from build123d import *

# Parameters (mm, degrees)
SKETCH1_W            = 350
SKETCH1_H            = 250
SKETCH1_W_2          = 329.63
SKETCH1_H_2          = 229.64
BOSS_EXTRUDE2_DEPTH  = 30
SKETCH1_3_W          = 329.63
SKETCH1_3_H          = 229.64
BOSS_EXTRUDE3_DEPTH  = 3.3
FILLET1_R            = 10
SKETCH3_W            = 40
SKETCH3_H            = 60
BOSS_EXTRUDE4_DEPTH  = 10
FILLET3_R            = 10
FILLET4_R            = 10
FILLET3_OF_MIRROR3_R = 10
FILLET4_OF_MIRROR3_R = 10
FILLET5_START        = 25.0000001
FILLET5_DEPTH        = 4.9999999
FILLET5_START_2      = 14.9999999
FILLET5_2_DEPTH      = 10.0000002
FILLET5_START_3      = -155
FILLET5_3_DEPTH      = 310


with BuildPart() as part:
    # Sketch1 → Boss-Extrude2 (new body)
    with BuildSketch(Plane(origin=(0, 0, 0), x_dir=(1, 0, 0), z_dir=(0, 1, 0))):
        Rectangle(SKETCH1_W, SKETCH1_H)
        Rectangle(SKETCH1_W_2, SKETCH1_H_2, mode=Mode.SUBTRACT)
    extrude(amount=BOSS_EXTRUDE2_DEPTH)

    # Sketch1<3> → Boss-Extrude3 (add)
    with BuildSketch(Plane(origin=(0, 0, 0), x_dir=(1, 0, 0), z_dir=(0, 1, 0))):
        Rectangle(SKETCH1_3_W, SKETCH1_3_H)
    extrude(amount=BOSS_EXTRUDE3_DEPTH)

    # Fillet1
    fillet1_edges = [part.edges().sort_by_distance(p)[0] for p in [
        (0, 0, -125),
        (175, 0, 0),
        (0, 0, 125),
        (-175, 0, 0),
        (-175, 15, -125),
        (175, 15, -125),
        (175, 15, 125),
        (-175, 15, 125),
    ]]
    fillet(fillet1_edges, radius=FILLET1_R)

    # Sketch3 → Boss-Extrude4 (add)
    with BuildSketch(Plane.XY.offset(125)):
        with Locations((-124.4, 45)):
            Rectangle(SKETCH3_W, SKETCH3_H)
    boss_extrude4 = extrude(amount=BOSS_EXTRUDE4_DEPTH)

    # Fillet3
    fillet3_edges = [part.edges().sort_by_distance(p)[0] for p in [
        (-124.4, 15, 135),
    ]]
    fillet(fillet3_edges, radius=FILLET3_R - 0.0001)  # a hair under: the kernel refuses the full size

    # Fillet4
    fillet4_edges = [part.edges().sort_by_distance(p)[0] for p in [
        (-124.4, 75, 135),
        (-104.4, 75, 130),
        (-144.4, 75, 130),
    ]]
    fillet(fillet4_edges, radius=FILLET4_R - 0.0001)  # a hair under: the kernel refuses the full size

    # Mirror3: Boss-Extrude4 across plane
    add(boss_extrude4.mirror(Plane.XY))

    # Fillet3 of Mirror3
    fillet3_of_mirror3_edges = [part.edges().sort_by_distance(p)[0] for p in [
        (-124.4, 15, -135),
    ]]
    fillet(fillet3_of_mirror3_edges, radius=FILLET3_OF_MIRROR3_R - 0.0001)  # a hair under: the kernel refuses the full size

    # Fillet4 of Mirror3
    fillet4_of_mirror3_edges = [part.edges().sort_by_distance(p)[0] for p in [
        (-124.4, 75, -135),
        (-104.4, 75, -130),
        (-144.4, 75, -130),
    ]]
    fillet(fillet4_of_mirror3_edges, radius=FILLET4_OF_MIRROR3_R - 0.0001)  # a hair under: the kernel refuses the full size

    # Mirror4: read off the stored shape, not the designer's step
    # Mirror4: part across plane


with BuildPart() as part_1:
    add(part.part)
    add(part.part.mirror(Plane(origin=(0, 0, 0), x_dir=(0, 0, 1), z_dir=(1, 0, 0))))

    # Fillet5: read off the stored shape, not the designer's step
    # Fillet5 outline → Fillet5 (add)
    with BuildSketch(Plane(origin=(0, 0, 0), x_dir=(1, 0, 0), z_dir=(0, 1, 0)).offset(FILLET5_START)):
        with BuildLine():
            Line((104.4, 125), (104.4, 135))
            ThreePointArc((104.4, 135), (101.471067812, 127.928932188), (94.4, 125))
            Line((94.4, 125), (104.4, 125))
        make_face()
        with BuildLine():
            Line((144.4, 135), (144.4, 125))
            Line((144.4, 125), (154.4, 125))
            ThreePointArc((154.4, 125), (147.328932188, 127.928932188), (144.4, 135))
        make_face()
        with BuildLine():
            Line((-154.4, 125), (-144.4, 125))
            Line((-144.4, 125), (-144.4, 135))
            ThreePointArc((-144.4, 135), (-147.328932188, 127.928932188), (-154.4, 125))
        make_face()
        with BuildLine():
            Line((-104.4, 125), (-94.4, 125))
            ThreePointArc((-94.4, 125), (-101.471067812, 127.928932188), (-104.4, 135))
            Line((-104.4, 135), (-104.4, 125))
        make_face()
        with BuildLine():
            Line((-144.4, -135), (-144.4, -125))
            Line((-144.4, -125), (-154.4, -125))
            ThreePointArc((-154.4, -125), (-147.328932188, -127.928932188), (-144.4, -135))
        make_face()
        with BuildLine():
            ThreePointArc((-104.4, -135), (-101.471067812, -127.928932188), (-94.4, -125))
            Line((-94.4, -125), (-104.4, -125))
            Line((-104.4, -125), (-104.4, -135))
        make_face()
        with BuildLine():
            Line((154.4, -125), (144.4, -125))
            Line((144.4, -125), (144.4, -135))
            ThreePointArc((144.4, -135), (147.328932188, -127.928932188), (154.4, -125))
        make_face()
        with BuildLine():
            ThreePointArc((94.4, -125), (101.471067812, -127.928932188), (104.4, -135))
            Line((104.4, -135), (104.4, -125))
            Line((104.4, -125), (94.4, -125))
        make_face()
    extrude(amount=FILLET5_DEPTH)

    # Fillet5 2 outline → Fillet5 2 (add)
    with BuildSketch(Plane(origin=(0, 0, 0), x_dir=(1, 0, 0), z_dir=(0, 1, 0)).offset(FILLET5_START_2)):
        with BuildLine():
            Line((104.4, 125), (104.4, 135))
            ThreePointArc((104.4, 135), (101.471067812, 127.928932188), (94.4, 125))
            Line((94.4, 125), (104.4, 125))
        make_face()
        with BuildLine():
            Line((144.4, 135), (144.4, 125))
            Line((144.4, 125), (154.4, 125))
            ThreePointArc((154.4, 125), (147.328932188, 127.928932188), (144.4, 135))
        make_face()
        with BuildLine():
            Line((-154.4, 125), (-144.4, 125))
            Line((-144.4, 125), (-144.4, 135))
            ThreePointArc((-144.4, 135), (-147.328932188, 127.928932188), (-154.4, 125))
        make_face()
        with BuildLine():
            Line((-104.4, 125), (-94.4, 125))
            ThreePointArc((-94.4, 125), (-101.471067812, 127.928932188), (-104.4, 135))
            Line((-104.4, 135), (-104.4, 125))
        make_face()
        with BuildLine():
            Line((-144.4, -135), (-144.4, -125))
            Line((-144.4, -125), (-154.4, -125))
            ThreePointArc((-154.4, -125), (-147.328932188, -127.928932188), (-144.4, -135))
        make_face()
        with BuildLine():
            ThreePointArc((-104.4, -135), (-101.471067812, -127.928932188), (-94.4, -125))
            Line((-94.4, -125), (-104.4, -125))
            Line((-104.4, -125), (-104.4, -135))
        make_face()
        with BuildLine():
            Line((154.4, -125), (144.4, -125))
            Line((144.4, -125), (144.4, -135))
            ThreePointArc((144.4, -135), (147.328932188, -127.928932188), (154.4, -125))
        make_face()
        with BuildLine():
            ThreePointArc((94.4, -125), (101.471067812, -127.928932188), (104.4, -135))
            Line((104.4, -135), (104.4, -125))
            Line((104.4, -125), (94.4, -125))
        make_face()
    extrude(amount=FILLET5_2_DEPTH)

    # Fillet5 3 outline → Fillet5 3 (cut)
    with BuildSketch(Plane.YZ.offset(FILLET5_START_3)):
        with BuildLine():
            Line((25, 135), (14.9999999, 135))
            Line((14.9999999, 135), (15, 125))
            ThreePointArc((15, 125), (17.928932188, 132.071067812), (25, 135))
        make_face()
        with BuildLine():
            ThreePointArc((25, -135), (17.928932188, -132.071067812), (15, -125))
            Line((15, -125), (14.9999999, -135))
            Line((14.9999999, -135), (25, -135))
        make_face()
    extrude(amount=FILLET5_3_DEPTH, mode=Mode.SUBTRACT)


solid = part_1.part
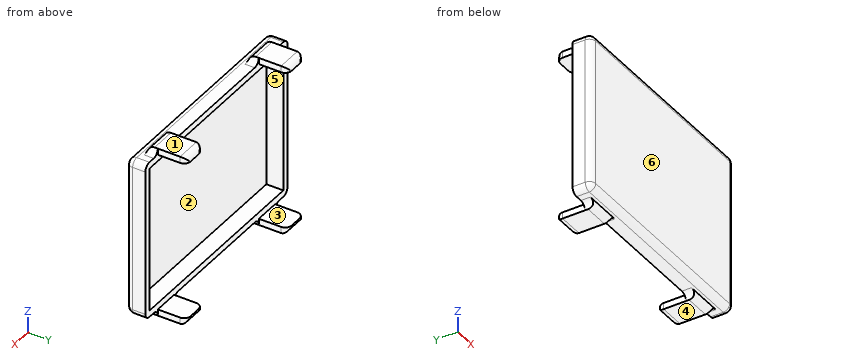
Geometry: final body of the model. Coordinates: model frame, mm. Face numbers are marked on the shaded views. A direction names the side the tool comes from. Coordinates: 2 decimals unless noted, no trailing zeros. Order: outer loops, then holes, each group sorted by start corner. A loop starts at its lowest first (then second) coordinate and runs counter-clockwise, first axis right, second up. Notation, with made-up numbers: M -27.5,10 L 22.5,10 A19 cw 22.5,21 Z; hole C 16,-15.5 d2. An arc over 180 degrees is marked long. One line per question, with ' | ' between items. Start each with the question number.
Item 1: Pin query (flat end, axial travel): pin 1 Ø3 at (y, z) = (44, -132.5) entering from -X; pin 2 Ø11 at (y, z) = (50.5, -127.5) entering from +X; pin 3 Ø10 at (x, y) = (115, 15.5) entering from +Z. Return the tip coordinate at first contact, or that it passes through.
Item 2: Cut plane C-C, the plane z = -26.5. Return the cut outline in (x, y) (3 decimals).
Item 3: Set-up query: the marked faces 1, 2 and 3. Return all of +Z, -Z, +X, -X, +Y, -Y with unobstructed straight access to the full face (end or side cutting, diameter ignored); none if empty.
Item 4: Cut plane A-A, the plane y = 37.5. Return the cut outline in (x, z), then the cut area to 3 significant figures.
Item 5: Draft query along Z for the marked faces 4, 5 and 6. Return one class per face: released by +Z, released by -Z, zero draft, split by the parting line, or undercut.
Item 6: Ray query, probe 1 along X at (y, z) = (28, 39.5) (3 decimals); probe 2 along Z at (x, y) = (126.5, 63); probe 3 along Z at (x, y) = (-72, 28.5). Return the intervals inside material, ascending. Write a range as [from, to].
Item 7: Cut plane D-D, the plane x = -1. Return the cut outline in (y, z).
A:
1) pin 1: stops at x = -144.4 | pin 2: stops at x = 144.4 | pin 3: stops at z = 133.93
2) outline: M -175,10 A10 ccw -165,0 L 165,0 A10 ccw 175,10 L 175,30 L 164.815,30 L 164.815,3.3 L -164.815,3.3 L -164.815,30 L -175,30 Z
3) face 1: +Z, +X, -X, +Y, -Y | face 2: +Y | face 3: +X, -X, +Y
4) outline: M -144.4,-135 L -104.4,-135 L -104.4,-125 L -144.4,-125 Z; M -144.4,125 L -104.4,125 L -104.4,135 L -144.4,135 Z; M 104.4,-135 L 144.4,-135 L 144.4,-125 L 104.4,-125 Z; M 104.4,125 L 144.4,125 L 144.4,135 L 104.4,135 Z | area: 1,600 mm2
5) face 4: released by -Z | face 5: undercut | face 6: zero draft
6) probe 1: x = [-175, -164.815], [164.815, 175] | probe 2: z = [-135, -125], [125, 135] | probe 3: z = [-125, -114.82], [114.82, 125]
7) outline: M 0,-115 A10 ccw 10,-125 L 30,-125 L 30,-114.82 L 3.3,-114.82 L 3.3,114.82 L 30,114.82 L 30,125 L 10,125 A10 ccw 0,115 Z
